Check sheet for the drawn part. Datum: minimum x, y, z corner. Units: mm. Round coordinates to 2 decimals unless told otherwise and drop trailing zeros. Write each loop counter-clockwise with the first axis right and the second up, starting at its lowest first coordinate (ties: lowest second). Pieces come first, ordered by that corner, then holes. Notation, with made-up numbers: (41.5, 46.5) - (62.5, 46.5) arc R6 ccw to (62.5, 53.5) - close; hole circle Ø7 at (29, 52.25). An arc over 180 degrees is marked (long way). Answer as a JSON object with one key per item and string values. Group by question number.
Item 1: Gauge pin test, flat ends, axial feed: P1, Ø1, axis at x = 1.5, y = 95.5, coming from the -Z side; P2, Ø1, axis at x = 1, y = 90.5, coming from the +Z side; P3, Ø0.6, axis at x = 1, z = 1, coming from the -Y side. Record the tip position at first contact, or that the pin passes through.
Item 2: Sectioned sample at B-B on x = 1.7. Count the separate pieces of the cut face and the enclosed holes in it, plus the area to 3 significant figures.
Item 3: Thickness scan on line 1 (Y direction, x = 0.9, z = 18); line 2 (Z direction, x = 0.55, y = 11.5). Record the ranges inside material, lowest first.
Item 4: Sectioned sample at A-A on z = 12.75. Record the boundary of the cut face in (x, y).
Item 5: Sectioned sample at C-C on y = 61. Record the boundary of the cut face in (x, z).
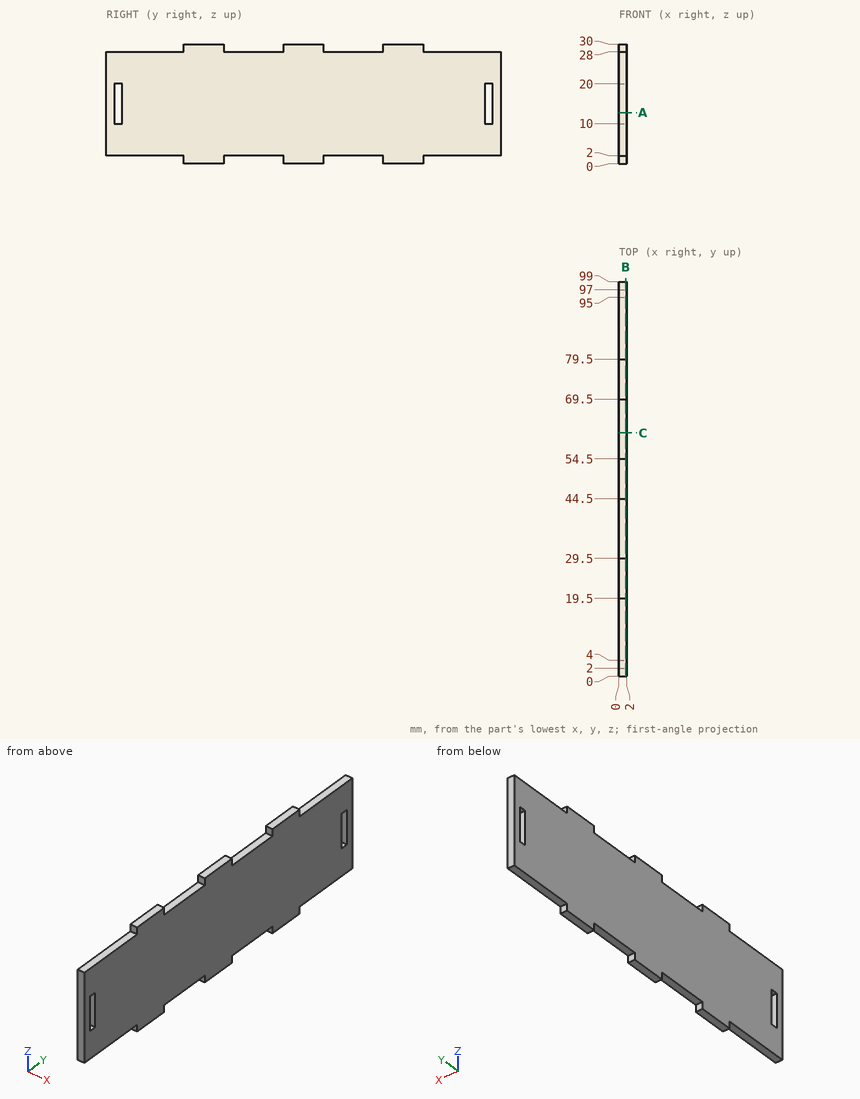
Completed:
{
 "1": {"P1": "z = 2", "P2": "z = 28", "P3": "y = 19.5"},
 "2": {"separate pieces": "1", "enclosed holes": "2", "area": "2,650 mm²"},
 "3": {"line 1": "0 to 2, 4 to 95, 97 to 99", "line 2": "2 to 28"},
 "4": {"outline": "(0, 0) - (2, 0) - (2, 2) - (0, 2) - close; (0, 4) - (2, 4) - (2, 95) - (0, 95) - close; (0, 97) - (2, 97) - (2, 99) - (0, 99) - close"},
 "5": {"outline": "(0, 2) - (2, 2) - (2, 28) - (0, 28) - close"}
}
